Design review of the part built by this model. Coordinates are the model's own, in mm. Face numbers are marked on the shaded views. A direction names the side the tool comes from. Round coordinates to 2 decimals unless told otherwise and drop trailing zeros. Order: outer loops, then holes, each group sorted by start corner. A loop starts at its lowest first (then second) coordinate and runs counter-clockwise, first axis right, second up. Notation, with made-up numbers: (3, -16.75) - (36, -16.75) arc R16 cw to (36, -9.75) - close; hole circle Ø6 at (-35.5, 49.5). An arc over 180 degrees is marked (long way). Use CSV: the item, a comma, the result in double quotes.
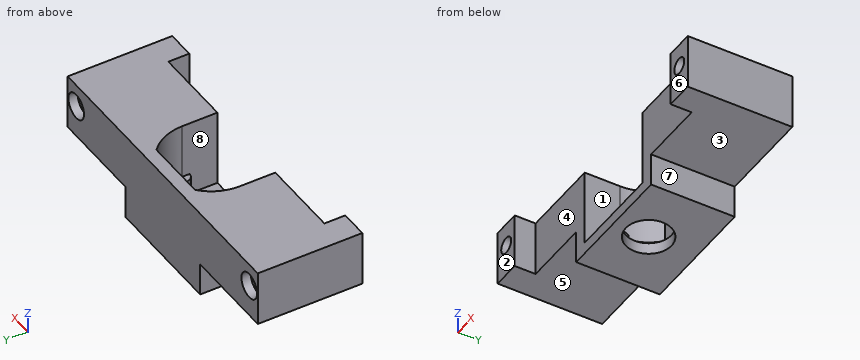
from build123d import *

# Parameters (mm, degrees)
BOSS_EXTRUDE2_DEPTH = 12
SKETCH2_W           = 12
SKETCH2_H           = 22.5
BOSS_EXTRUDE3_DEPTH = 6
SKETCH3_W           = 12
SKETCH3_H           = 22.5
BOSS_EXTRUDE4_DEPTH = 6
SKETCH4_R           = 1.75
CUT_EXTRUDE1_DEPTH  = 22.5
BOSS_EXTRUDE5_DEPTH = 4.65
SKETCH6_W           = 26.4
SKETCH6_H           = 18
SKETCH6_R           = 4.925
BOSS_EXTRUDE6_DEPTH = 2.5
SKETCH7_R           = 2.75
CUT_EXTRUDE2_DEPTH  = 2


with BuildPart() as part:
    # Sketch1 → Boss-Extrude2 (new body)
    with BuildSketch(Plane.XY):
        Polygon((0, 18), (0, 0), (17.3, 0), (17.3, 7.6), (17.3, 15.2), (20.697059459, 15.2), (34.302940541, 15.2), (37.7, 15.2), (37.7, 7.6), (37.7, 0), (55, 0), (55, 18), align=None)
        with BuildLine():
            Line((17.3, 15.2), (17.3, 7.6))
            ThreePointArc((17.3, 7.6), (18.187911257, 11.762331467), (20.697059459, 15.2))
            Line((20.697059459, 15.2), (17.3, 15.2))
        make_face()
        with BuildLine():
            Line((37.7, 15.2), (34.302940541, 15.2))
            ThreePointArc((34.302940541, 15.2), (36.812088743, 11.762331467), (37.7, 7.6))
            Line((37.7, 7.6), (37.7, 15.2))
        make_face()
    extrude(amount=BOSS_EXTRUDE2_DEPTH)

    # Sketch2 → Boss-Extrude3 (add)
    with BuildSketch(Plane.ZY):
        with Locations((6, 6.75)):
            Rectangle(SKETCH2_W, SKETCH2_H)
    extrude(amount=BOSS_EXTRUDE3_DEPTH)

    # Sketch3 → Boss-Extrude4 (add)
    with BuildSketch(Plane(origin=(55, 0, 0), x_dir=(0, 0, -1), z_dir=(1, 0, 0))):
        with Locations((-6, 6.75)):
            Rectangle(SKETCH3_W, SKETCH3_H)
    extrude(amount=BOSS_EXTRUDE4_DEPTH)

    # Sketch4 → Cut-Extrude1 (cut)
    with BuildSketch(Plane(origin=(0, 18, 0), x_dir=(1, 0, 0), z_dir=(0, 1, 0))):
        with Locations((-3, -7)):
            Circle(SKETCH4_R)
        with Locations((58, -7)):
            Circle(SKETCH4_R)
    extrude(amount=-CUT_EXTRUDE1_DEPTH, mode=Mode.SUBTRACT)

    # Sketch5 → Boss-Extrude5 (add)
    with BuildSketch(Plane(origin=(0, 0, 0), x_dir=(-1, 0, 0), z_dir=(0, 0, -1))):
        with BuildLine():
            Line((-37.7, 0), (-40.7, 0))
            Line((-40.7, 0), (-40.7, 18))
            Line((-40.7, 18), (-14.3, 18))
            Line((-14.3, 18), (-14.3, 0))
            Line((-14.3, 0), (-17.3, 0))
            Line((-17.3, 0), (-17.3, 6))
            ThreePointArc((-17.3, 6), (-18.898767331, 7.537206525), (-17.425490196, 9.195071224))
            ThreePointArc((-17.425490196, 9.195071224), (-18.543054375, 12.47986937), (-20.697059459, 15.2))
            Line((-20.697059459, 15.2), (-34.302940541, 15.2))
            ThreePointArc((-34.302940541, 15.2), (-36.456945625, 12.47986937), (-37.574509804, 9.195071224))
            ThreePointArc((-37.574509804, 9.195071224), (-36.101232669, 7.537206525), (-37.7, 6))
            Line((-37.7, 6), (-37.7, 0))
        make_face()
    extrude(amount=BOSS_EXTRUDE5_DEPTH)

    # Sketch6 → Boss-Extrude6 (add)
    with BuildSketch(Plane(origin=(0, 0, -4.65), x_dir=(-1, 0, 0), z_dir=(0, 0, -1))):
        with Locations((-27.5, 9)):
            Rectangle(SKETCH6_W, SKETCH6_H)
        with Locations((-27.5, 7.537206525)):
            Circle(SKETCH6_R, mode=Mode.SUBTRACT)
    extrude(amount=BOSS_EXTRUDE6_DEPTH)

    # Sketch7 → Cut-Extrude2 (cut)
    with BuildSketch(Plane(origin=(0, 18, 0), x_dir=(1, 0, 0), z_dir=(0, 1, 0))):
        with Locations((-3, -7)):
            Circle(SKETCH7_R)
        with Locations((58, -7)):
            Circle(SKETCH7_R)
    extrude(amount=-CUT_EXTRUDE2_DEPTH, mode=Mode.SUBTRACT)


solid = part.part
1) To check wall thickness, follow L1, parallel to X at y = 0.5, z = 7; L2, parallel to X at y = 17.25, z = 7; L3, parallel to Z at x = 58, y = 0. State the ranges of each line that lie inside material, in increasing order. Write a range as from..to.
Data:
L1,"x = -6..-4.75, -1.25..17.3, 37.7..56.25, 59.75..61"
L2,"x = -6..-5.75, -0.25..55.25, 60.75..61"
L3,"z = 0..5.25, 8.75..12"
2) We need section C-C (z = -3.25). Give the boundary of the cut face in (x, y).
Data:
outline,"(14.3, 0) - (17.3, 0) - (17.3, 6) arc R1.6 ccw to (17.43, 9.2) arc R10.2 cw to (20.7, 15.2) - (34.3, 15.2) arc R10.2 cw to (37.57, 9.2) arc R1.6 ccw to (37.7, 6) - (37.7, 0) - (40.7, 0) - (40.7, 18) - (14.3, 18) - close"
3) We need section B-B (z = 6). Give the number of separate pieces and of enclosed holes in the cut face, then the cut area to 3 significant figures.
Data:
separate pieces,"3"
enclosed holes,"0"
area,"828 mm2"
4) We need section A-A (x = 30). Give the boundary of the cut face in (y, z).
Data:
outline,"(0, -7.15) - (3.29, -7.15) - (3.29, -4.65) - (0, -4.65) - close; (11.78, -7.15) - (18, -7.15) - (18, 12) - (15.2, 12) - (15.2, -4.65) - (11.78, -4.65) - close"
5) We need section D-D (x = 53). Give the boundary of the cut face in (y, z), then the cut area to 3 significant figures.
Data:
outline,"(0, 0) - (18, 0) - (18, 12) - (0, 12) - close"
area,"216 mm2"
6) The part is to be moulded in two halves that separate along X. For the marked faces 6, 7 and 8, say which applies: +X half, -X half, draft (parallel to the pull), parting line (faces both ways), or undercut.
Data:
face 6,"draft"
face 7,"+X half"
face 8,"undercut"
7) Insertion check: pin 1 Ø2 at (y, z) = (13, -5.5) entering from -X; pin 2 Ø4 at (x, z) = (28, 0.5) entering from -Y; pin 3 Ø6 at (x, y) = (46, 6.5) entering from -Z; pin 4 Ø6 at (x, y) = (27.5, 7.54) entering from +Z. Each pin has a flat end and moves straight along its axis. Give the tip position at first contact, or say it passes through.
Data:
pin 1,"stops at x = 14.3"
pin 2,"stops at y = 15.2"
pin 3,"stops at z = 0"
pin 4,"passes through"
8) For the marked faces 1, 2, 3, 4 and 5, list the 3-axis set-ups (+Z, -Z, +X, -X, +Y, -Y) from which the entire face can be reached by the end or side of a thin tool; tool diameter is ignored.
Data:
face 1,"+Z, -Y"
face 2,"+Z, -Z, +X, -X, -Y"
face 3,"-Z, +X, +Y, -Y"
face 4,"+Z, -Z, -Y"
face 5,"-Z, -X, +Y, -Y"
